```python
from build123d import *

# Parameters (mm, degrees)
SKETCH_1_W      = 5
SKETCH_1_H      = 5
SKETCH_1_R      = 1.1
EXTRUDE_1_DEPTH = 2
SKETCH_2_W      = 5
SKETCH_2_H      = 3
EXTRUDE_2_DEPTH = 35
SKETCH_3_W      = 5
SKETCH_3_H      = 5
SKETCH_3_R      = 0.75
EXTRUDE_3_DEPTH = 3


with BuildPart() as part:
    # 草图1 → 凸台-拉伸1 (new body)
    with BuildSketch(Plane(origin=(0, 0, 0), x_dir=(1, 0, 0), z_dir=(0, 1, 0))):
        Rectangle(SKETCH_1_W, SKETCH_1_H)
        with Locations(Location((0, 0, 0), (0, 0, 270))):
            Circle(SKETCH_1_R, mode=Mode.SUBTRACT)
    extrude(amount=EXTRUDE_1_DEPTH)

    # 草图2 → 凸台-拉伸2 (add)
    with BuildSketch(Plane.XZ):
        with Locations((0, 4)):
            Rectangle(SKETCH_2_W, SKETCH_2_H)
    extrude(amount=-EXTRUDE_2_DEPTH)

    # 草图3 → 凸台-拉伸3 (add)
    with BuildSketch(Plane(origin=(0, 35, 0), x_dir=(1, 0, 0), z_dir=(0, 1, 0))):
        with Locations((0, -8)):
            Rectangle(SKETCH_3_W, SKETCH_3_H)
        with Locations(Location((0, -8, 0), (0, 0, 270))):
            Circle(SKETCH_3_R, mode=Mode.SUBTRACT)
    extrude(amount=-EXTRUDE_3_DEPTH)


solid = part.part
```
Verification items for the finished model (mm, model axes). A direction names the side the tool comes from. Round coordinates to 2 decimals unless told otherwise and drop trailing zeros. Write each loop counter-clockwise with the first axis right and the second up, starting at its lowest first coordinate (ties: lowest second). Pieces come first, ordered by that corner, then holes. Notation, with made-up numbers: (78.5, 1.25) - (116.5, 1.25) arc R34 ccw to (116.5, 33.25) - close; hole circle Ø4 at (-21.5, 37). An arc over 180 degrees is marked (long way). Answer as a JSON object with one key per item and string values. Group by question number.
Q1. Tool access check on faces 4 (the flat face through (-1, 32, 7)), 5 (the flat face through (2.5, 19, 4)). Record the directions out of +Z, -Z, +X, -X, +Y, -Y that give a thin tool (end or side, any length) a straight path to the whole face; none if there is none.
Q2. Section check D-D, the plane z = 8. Enter the section's corners in (x, y), plus the area to 3 significant figures.
Q3. Go/stop test with a flat-tipped pin: pin 1 Ø3 at (x, z) = (0, 0) entering from +Y. Record where the tip stops, or that it passes through.
Q4. Section check B-B, the plane x = 0. Enter the section's corners in (y, z).
Q5. Mould release check, pull along Y, two halves, no side actions. Record for faces 1 (the flat face through (0, 0, 2)), 2 (the flat face through (0, 18, 2.5)), 3 (the flat face through (-1, 2, -1)): released by +Y, released by -Y, zero draft, split by the parting line, or undercut.
Q6. Section check A-A, the plane z = 0. Enter the section's corners in (x, y).
Q7. Thickness scan on line 1 (X direction, y = 34.25, z = 8); line 2 (X direction, y = 0.8, z = 0); line 3 (Z direction, x = 1.45, y = 4). Record the ranges inside material, lowest first.
Q8. Section check C-C, the plane x = 1.8. Enter the section's corners in (y, z), plus the area to 3 significant figures.
Found:
{
 "1": {"face 4": "+Z, +X, -X, -Y", "face 5": "+Z, -Z, +X, +Y, -Y"},
 "2": {"outline": "(-2.5, 32) - (-0.75, 32) - (-0.75, 35) - (-2.5, 35) - close; (0.75, 32) - (2.5, 32) - (2.5, 35) - (0.75, 35) - close", "area": "10.5 mm^2"},
 "3": {"pin 1": "stops at y = 2"},
 "4": {"outline": "(0, -2.5) - (2, -2.5) - (2, -1.1) - (0, -1.1) - close; (0, 1.1) - (2, 1.1) - (2, 2.5) - (35, 2.5) - (35, 7.25) - (32, 7.25) - (32, 5.5) - (0, 5.5) - close; (32, 8.75) - (35, 8.75) - (35, 10.5) - (32, 10.5) - close"},
 "5": {"face 1": "released by -Y", "face 2": "zero draft", "face 3": "released by +Y"},
 "6": {"outline": "(-2.5, 0) - (-1.1, 0) - (-1.1, 2) - (-2.5, 2) - close; (1.1, 0) - (2.5, 0) - (2.5, 2) - (1.1, 2) - close"},
 "7": {"line 1": "x = -2.5 to -0.75, 0.75 to 2.5", "line 2": "x = -2.5 to -1.1, 1.1 to 2.5", "line 3": "z = 2.5 to 5.5"},
 "8": {"outline": "(0, -2.5) - (2, -2.5) - (2, 2.5) - (35, 2.5) - (35, 10.5) - (32, 10.5) - (32, 5.5) - (0, 5.5) - close", "area": "130 mm^2"}
}
